Build history of the part. All positions in model axes, mm. A direction names the side the tool comes from. Round coordinates to 2 decimals unless told otherwise and drop trailing zeros. Order: outer loops, then holes, each group sorted by start corner. A loop starts at its lowest first (then second) coordinate and runs counter-clockwise, first axis right, second up. Notation, with made-up numbers: (40, 51) -> (56, 51) arc R19 cw to (56, 61) -> close; hole circle Ø4 at (25.25, -29). An arc over 180 degrees is marked (long way). Write item = value, one per line.
Solid Edge part; units mm, degrees
sketch "Sketch1" plane through (0, 0, -20) normal (0, 0, -1) x (-1, 0, 0)
  line L0 (-67.0152, -63.9403) -> (-67.0152, -42.9403)
  line L1 (-67.0152, -42.9403) -> (-49.5152, -42.9403)
  line L2 (-49.5152, -42.9403) -> (-49.5152, 15.0597)
  line L3 (-49.5152, 15.0597) -> (-67.0152, 15.0597)
  line L4 (-67.0152, 15.0597) -> (-67.0152, 36.0597)
  line L5 (-67.0152, 36.0597) -> (-102.0152, 36.0597)
  line L6 (-102.0152, 36.0597) -> (-102.0152, 15.0597)
  line L7 (-102.0152, 15.0597) -> (-119.5152, 15.0597)
  line L8 (-119.5152, 15.0597) -> (-119.5152, -42.9403)
  line L9 (-119.5152, -42.9403) -> (-102.0152, -42.9403)
  line L10 (-102.0152, -42.9403) -> (-102.0152, -63.9403)
  line L11 (-102.0152, -63.9403) -> (-67.0152, -63.9403)
  circle A0 centre (-75.7833, -56.8959) radius 1.7228
  circle A1 centre (-93.2363, -56.8951) radius 1.741
  circle A2 centre (-93.247, 29.0153) radius 1.735
  circle A3 centre (-75.7554, 29.0254) radius 1.7262
extrude "Protrusion1" add sketch "Sketch1" along normal blind 8
sketch "Sketch2" plane through (84.5152, -13.9403, -20) normal (0, 0, 1) x (0, -1, 0)
  arc A0 (-41.5739, 9.7812) -> (-44.4734, 9.5724) centre (-42.9556, 8.7318) ccw
  arc A1 (-44.4734, 9.5724) -> (-41.5739, 9.7812) centre (-42.9548, 8.7211) ccw
  line L0 (-38.7893, 17.5) -> (-38.7893, -17.5)
  line L1 (-38.7893, -17.5) -> (-50, -17.5)
  line L2 (-50, -17.5) -> (-50, 17.5)
  line L3 (-50, 17.5) -> (-38.7893, 17.5)
  arc A2 (-44.5058, -7.9803) -> (-41.2822, -9.1415) centre (-42.9657, -8.7598) ccw
  arc A3 (-41.2822, -9.1415) -> (-44.5058, -7.9803) centre (-42.9556, -8.7318) ccw
extrude "ExtrudedCutout_1" add sketch "Sketch2" along normal blind 10
fillet "Round_1" radius 5 1 edges at (84.5152, 36.0597, -28)
mirror "Mirror1" about plane through (84.5152, -13.9403, -24) normal (0, -1, 0) of "ExtrudedCutout_1"
fillet "Round1" radius 5 1 edges at (84.5152, -63.9403, -28)
sketch "Sketch3" plane through (84.5152, -13.9403, -28) normal (0, 0, -1) x (-1, 0, 0)
  circle A0 centre (-8.7318, 42.9556) radius 3.15
  circle A1 centre (-8.7318, 42.9556) radius 1.735
  circle A2 centre (8.7598, 42.9657) radius 3.15
  circle A3 centre (8.7598, 42.9657) radius 1.7262
  circle A4 centre (-8.7211, -42.9548) radius 3.15
  circle A5 centre (-8.7211, -42.9548) radius 1.741
  circle A6 centre (8.7318, -42.9556) radius 3.15
  circle A7 centre (8.7318, -42.9556) radius 1.7228
extrude "ExtrudedCutout_2" cut sketch "Sketch3" against normal blind 10
sketch "Sketch4" plane through (110.7652, 15.0597, -24) normal (0, 1, 0) x (0, 0, -1)
  arc A0 (4, 49.1033) -> (4, 55.1033) centre (4, 52.1033) cw
  line L0 (4, 55.1033) -> (4, 49.1033)
  arc A1 (4, -3) -> (4, 3) centre (4, 0) cw
  line L1 (4, 3) -> (4, -3)
extrude "ExtrudedCutout_3" cut sketch "Sketch4" against normal blind 119
Q1. Cut at A-A, the plane z = -26. List the corners of the cut face in (x, y).
Check values:
outline = (49.52, -42.94) -> (56.43, -42.94) -> (56.43, 15.06) -> (49.52, 15.06) -> close; (60.9, -42.94) -> (67.02, -42.94) -> (67.02, -62.94) -> (102.02, -62.94) -> (102.02, -42.94) -> (108.53, -42.94) -> (108.53, 15.06) -> (102.02, 15.06) -> (102.02, 35.06) -> (67.02, 35.06) -> (67.02, 15.06) -> (60.9, 15.06) -> close; (113, -42.94) -> (119.52, -42.94) -> (119.52, 15.06) -> (113, 15.06) -> close; hole circle Ø6.3 at (75.76, 29.03); hole circle Ø6.3 at (75.78, -56.9); hole circle Ø6.3 at (93.24, -56.9); hole circle Ø6.3 at (93.25, 29.02)
Q2. Probe probe 1 along Y at (x, z) = (86.5, -11); probe 2 along X at (y, z) = (1, -25.5); probe 3 along Y at (x, z) = (74, -26.75). List the from-to ranges inside material, lowest first.
Check values:
probe_1 = -63.94 to -52.73, 24.85 to 36.06
probe_2 = 49.52 to 57, 60.32 to 109.11, 112.42 to 119.52
probe_3 = -62.25 to -59.49, -54.3 to 26.41, 31.64 to 34.37
Q3. Which spindle directions (+Z, -Z, +X, -X, +Y, -Y) get a long thin tool onto all of the face, cutting with end or side? Do faces 4 (the face through (102.015, -56, -21)), 5 (the face through (67.015, -56, -21)), 6 (the face through (91.89, 27.66, -18)), 7 (the face through (85, 24.849, -15)), 8 (the face through (67.015, 28, -21)). Say none if no direction does.
Check values:
face_4 = +Z, -Z, +X, -Y
face_5 = +Z, -Z, -X, -Y
face_6 = -Z
face_7 = +Z, +X, -X
face_8 = +Z, -Z, -X, +Y
Q4. Cut at B-B, the plane y = -27. List the corners of the cut face in (x, z), and give its area (3 significant figures).
Check values:
outline = (49.52, -28) -> (55.66, -28) arc R3 cw to (61.66, -28) -> (107.77, -28) arc R3 cw to (113.77, -28) -> (119.52, -28) -> (119.52, -20) -> (49.52, -20) -> close
area = 532 mm²
Q5. Flat gauge pins, fed straight in: pin 1 (9 mm diameter, centred on x = 107, z = -24.5, fed in from +Y); pin 2 (8 mm diameter, centred on x = 80.5, y = -33, fed in from +Z); pin 3 (4 mm diameter, centred on x = 57.5, z = -23.5, fed in from -Y). Where does each tip first touch, or does it go through?
Check values:
pin_1 = 15.06
pin_2 = -20
pin_3 = -42.94
Q6. Cut at C-C, the plane x = 80. List the corners of the cut face in (y, z), and give its area (3 significant figures).
Check values:
outline = (-63.94, -23) arc R5 ccw to (-58.94, -28) -> (31.06, -28) arc R5 ccw to (36.06, -23) -> (36.06, -10) -> (24.85, -10) -> (24.85, -20) -> (-52.73, -20) -> (-52.73, -10) -> (-63.94, -10) -> close
area = 1,010 mm²
Q7. Mould opens along Y. For faces 1 (the face through (110.7, -13.5, -25)), 2 (the face through (111, -42.94, -24)), 3 (the face through (77.416, 28.465, -14.056)) say: released by +Y, released by -Y, zero draft, split by the parting line, or undercut.
Check values:
face_1 = zero draft
face_2 = released by -Y
face_3 = undercut
